Input: part model. Units: mm. Frame: model coordinates. A direction names the side the tool comes from. Coordinates: 2 decimals unless noted, no trailing zeros. Loops run counter-clockwise (first coordinate to the right, second up) from the corner with the lowest first, then second, coordinate; pieces in that order, holes last.
(1) Section A-A, the plane z = 1.7. Return loops of the section in (x, y), then the cut area to 3 significant figures.
(2) Set-up query: faces 1 (the face through (29, 68.681, 1)), 2 (the face through (11, 94.181, 1)), 3 (the face through (12.065, 9, 1)), 4 (the face through (15.984, 91.435, 0.986)). Return all of +Z, -Z, +X, -X, +Y, -Y with unobstructed straight access to the full face (end or side cutting, diameter ignored); none if empty.
(3) Section B-B, the plane y = 53. Return loops of the section in (x, z).
(4) Contact query for flat-ended pins moving along their axis: P1, Ø0.6, axis at x = 13, z = 1, coming from the -Y side; P2, Ø1.2, axis at x = 10.5, z = 1, coming from the +Y side; P3, Ø1, axis at x = 36, z = 1, coming from the +Y side. Output: stop coordinate, or through.
(5) Line query: L1, parallel to Y at x = 11.5, z = 0.8; L2, parallel to Y at x = 31, z = 0.6; L3, parallel to X at y = 80.5, z = 0.7. Output: solid intervals per line, ascending.
(6) Section C-C, the plane x = 26. Return loops of the section in (y, z), then the cut area to 3 significant figures.
(7) Mould query, pull axis Y, two halves, no side actions, for faces 5 (the face through (11, 5.298, 1)), 6 (the face through (18.59, 86.03, 0.99)), 7 (the face through (11.565, 96, 1)), 8 (the face through (13.34, 94.54, 0.99)). Classes: released by +Y, released by -Y, zero draft, split by the parting line, or undercut.
```python
from build123d import *

# Parameters (mm, degrees)
SKETCH_1_R      = 0.5
EXTRUDE_1_DEPTH = 2


with BuildPart() as part:
    # 草图1 → 凸台-拉伸1 (new body)
    with BuildSketch(Plane.XY):
        with BuildLine():
            Line((15.072355278, 90.9902121), (11.565386103, 98.180564471))
            Line((11.565386103, 98.180564471), (11.565386103, 94.180564471))
            Line((11.565386103, 94.180564471), (10.065386103, 94.180564471))
            Line((10.065386103, 94.180564471), (10.065386103, 5.297847711))
            Line((10.065386103, 5.297847711), (12.065386103, 5.297847711))
            Line((12.065386103, 5.297847711), (12.065386103, 13.547847711))
            Line((12.065386103, 13.547847711), (14.065386103, 13.547847711))
            Line((14.065386103, 13.547847711), (14.065386103, 5.297847711))
            Line((14.065386103, 5.297847711), (14.686363295, 5.297847711))
            Line((14.686363295, 5.297847711), (21.506195844, 68.680564471))
            Line((21.506195844, 68.680564471), (37.065386103, 68.680564471))
            ThreePointArc((37.065386103, 68.680564471), (39.053255495, 70.460620657), (37.502605679, 72.632189189))
            Line((37.502605679, 72.632189189), (22.373010944, 76.021649743))
            Line((22.373010944, 76.021649743), (21.07399479, 78.685027553))
            Line((21.07399479, 78.685027553), (17.702582158, 85.597447823))
            Line((17.702582158, 85.597447823), (19.500170251, 86.474190116))
            Line((19.500170251, 86.474190116), (16.86994337, 91.866954394))
            Line((16.86994337, 91.866954394), (15.072355278, 90.9902121))
        make_face()
        with Locations((37.065386103, 70.680564471)):
            Circle(SKETCH_1_R, mode=Mode.SUBTRACT)
    extrude(amount=EXTRUDE_1_DEPTH)


solid = part.part
```
Report:
1. outline: (10.07, 5.3) - (12.07, 5.3) - (12.07, 13.55) - (14.07, 13.55) - (14.07, 5.3) - (14.69, 5.3) - (21.51, 68.68) - (37.07, 68.68) arc R2 ccw to (37.5, 72.63) - (22.37, 76.02) - (17.7, 85.6) - (19.5, 86.47) - (16.87, 91.87) - (15.07, 90.99) - (11.57, 98.18) - (11.57, 94.18) - (10.07, 94.18) - close; hole circle Ø1 at (37.07, 70.68)
1. area: 831 mm2
2. face 1: +Z, -Z, +X, -Y
2. face 2: +Z, -Z, -X, +Y
2. face 3: +Z, -Z, -Y
2. face 4: +Z, -Z, +Y
3. outline: (10.07, 0) - (19.82, 0) - (19.82, 2) - (10.07, 2) - close
4. P1: stops at y = 13.55
4. P2: stops at y = 94.18
4. P3: stops at y = 73.08
5. L1: y = 5.3 to 94.18
5. L2: y = 68.68 to 74.09
5. L3: x = 10.07 to 20.19
6. outline: (68.68, 0) - (75.21, 0) - (75.21, 2) - (68.68, 2) - close
6. area: 13.1 mm2
7. face 5: released by -Y
7. face 6: undercut
7. face 7: zero draft
7. face 8: released by +Y
